The model under review builds one solid part; all positions refer to its coordinate system, in mm. Face numbers are marked on the shaded views. Round coordinates to 2 decimals unless told otherwise and drop trailing zeros. Write each loop counter-clockwise with the first axis right and the second up, starting at its lowest first coordinate (ties: lowest second). Pieces come first, ordered by that corner, then holes.
Item 1: Add section C-C (z = 30.5). Give the boundary of the cut face in (x, y), plus the area to 3 significant figures.
Item 2: Draft analysis for pull direction Z (two halves, no side actions). For the marked faces 1, 2 and 3, state which applies: +Z half, -Z half, draft (parallel to the pull), parting line (faces both ways), or undercut.
Item 3: Add section B-B (x = 34.5). Give the boundary of the cut face in (y, z).
Item 4: To check wall thickness, follow L1, parallel to Z at x = 73, y = -2.25; L2, parallel to X at y = -3, z = 8; L3, parallel to Y at x = 53, z = 40. State the ranges of each line that lie inside material, in increasing order.
Item 5: Add section A-A (y = -3.5). Give the boundary of the cut face in (x, z), plus the area to 3 significant figures.
Item 6: Clearance check with a flat-ended pin moving along its axis: pin 1 Ø15.5 at (x, z) = (42, 14) entering from -Y. State where the tip first meets the part, or that it passes through.
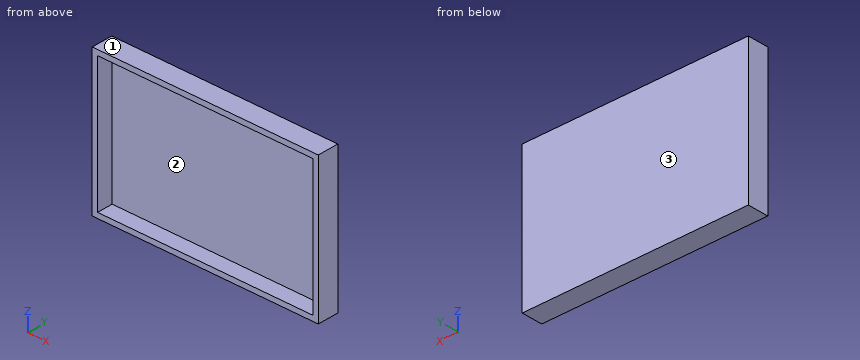
```python
from build123d import *

# Parameters (mm, degrees)
SKETCH1_W           = 81.5
SKETCH1_H           = 51
BOSS_EXTRUDE1_DEPTH = 2
SKETCH2_W           = 85.5
SKETCH2_H           = 55
SKETCH2_W_2         = 81.5
SKETCH2_H_2         = 51
BOSS_EXTRUDE2_DEPTH = 8


with BuildPart() as part:
    # Sketch1 → Boss-Extrude1 (new body)
    with BuildSketch(Plane(origin=(0, 0, 0), x_dir=(1, 0, 0), z_dir=(0, 1, 0))):
        with Locations((40.75, -25.5)):
            Rectangle(SKETCH1_W, SKETCH1_H)
    extrude(amount=BOSS_EXTRUDE1_DEPTH)

    # Sketch2 → Boss-Extrude2 (add)
    with BuildSketch(Plane(origin=(0, 2, 0), x_dir=(1, 0, 0), z_dir=(0, 1, 0))):
        with Locations((40.75, -25.5)):
            Rectangle(SKETCH2_W, SKETCH2_H)
        with Locations((40.75, -25.5)):
            Rectangle(SKETCH2_W_2, SKETCH2_H_2, mode=Mode.SUBTRACT)
    extrude(amount=-BOSS_EXTRUDE2_DEPTH)


solid = part.part
```
Numbers:
1. outline: (-2, -6) - (0, -6) - (0, 0) - (81.5, 0) - (81.5, -6) - (83.5, -6) - (83.5, 2) - (-2, 2) - close
1. area: 195 mm2
2. face 1: +Z half
2. face 2: undercut
2. face 3: draft
3. outline: (-6, -2) - (2, -2) - (2, 53) - (-6, 53) - (-6, 51) - (0, 51) - (0, 0) - (-6, 0) - close
4. L1: z = -2 to 0, 51 to 53
4. L2: x = -2 to 0, 81.5 to 83.5
4. L3: y = 0 to 2
5. outline: (-2, -2) - (83.5, -2) - (83.5, 53) - (-2, 53) - close; hole (0, 0) - (81.5, 0) - (81.5, 51) - (0, 51) - close
5. area: 546 mm2
6. pin 1: stops at y = 0
